Here's the drawing with two shaded views (mm, measured from the low corner). I have some questions. Coordinates: 2 decimals unless noted, no trailing zeros. Order: outer loops, then holes, each group sorted by start corner. A loop starts at its lowest first (then second) coordinate and runs counter-clockwise, first axis right, second up. Notation, with made-up numbers: (71.25, -27) - (84.25, -27) arc R21 cw to (84.25, -7) - close; hole circle Ø9 at (73.5, 44.25). An arc over 180 degrees is marked (long way). Answer as a JSON object with one key per item and string values. Group by question number.
(1) Imagine slicing it at B-B, the plane z = 1.2. Write out the boundary of the cut face in (x, y), and give its area (3 significant figures).
(2) Imagine slicing it at A-A, the plane x = 9.7. Write out the boundary of the cut face in (y, z).
(3) Imagine slicing it at C-C, the plane y = 13.5. Write out the boundary of the cut face in (x, z).
(4) Will this pin go through, and if not, where does the flat tip stop? P1, Ø4, axis at x = 135.7, y = 7.5, coming from the +Z side.
(5) Please list where these lines run through material, in increasing order: probe 1 along X at (y, z) = (7.25, 1.15); probe 2 along X at (y, z) = (6, 1.8); probe 3 along Y at (x, z) = (9.7, 0.7).
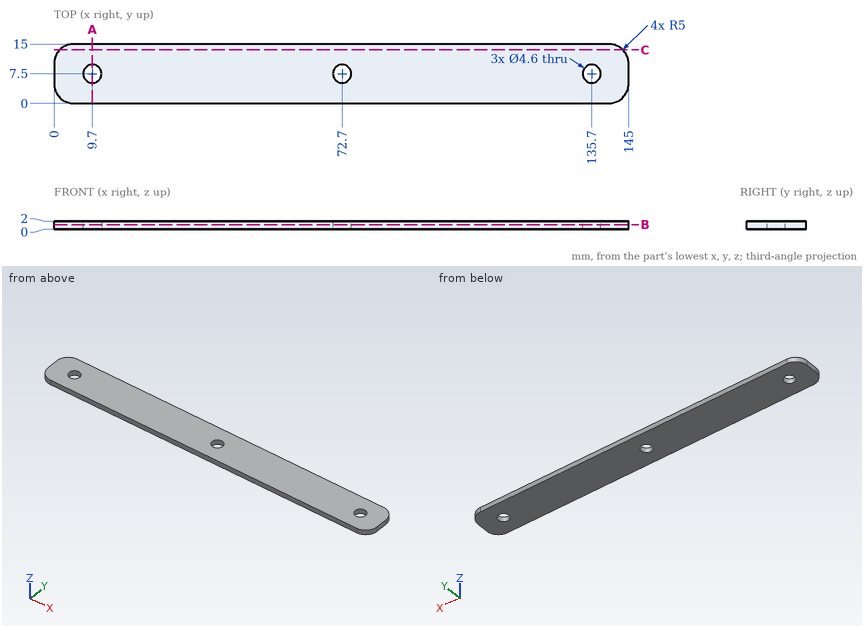
Result set:
{
 "1": {"outline": "(0, 5) arc R5 ccw to (5, 0) - (140, 0) arc R5 ccw to (145, 5) - (145, 10) arc R5 ccw to (140, 15) - (5, 15) arc R5 ccw to (0, 10) - close; hole circle Ø4.6 at (9.7, 7.5); hole circle Ø4.6 at (72.7, 7.5); hole circle Ø4.6 at (135.7, 7.5)", "area": "2,100 mm^2"},
 "2": {"outline": "(0, 0) - (5.2, 0) - (5.2, 2) - (0, 2) - close; (9.8, 0) - (15, 0) - (15, 2) - (9.8, 2) - close"},
 "3": {"outline": "(1.43, 0) - (143.57, 0) - (143.57, 2) - (1.43, 2) - close"},
 "4": {"P1": "passes through"},
 "5": {"probe 1": "x = 0 to 7.41, 11.99 to 70.41, 74.99 to 133.41, 137.99 to 145", "probe 2": "x = 0 to 7.96, 11.44 to 70.96, 74.44 to 133.96, 137.44 to 145", "probe 3": "y = 0 to 5.2, 9.8 to 15"}
}
